Verification items for this drawing (mm, ordinates from the low corner). Round coordinates to 2 decimals unless told otherwise and drop trailing zeros. Loops run counter-clockwise (first coordinate to the right, second up) from the corner with the lowest first, then second, coordinate; pieces in that order, holes last. Notation, with made-up numbers: M -4.75,27 L 1.25,27 A25 ccw 1.25,59 Z; hole C 1,-40 d11. An arc over 180 degrees is marked long. Answer as CSV lines item,"result".
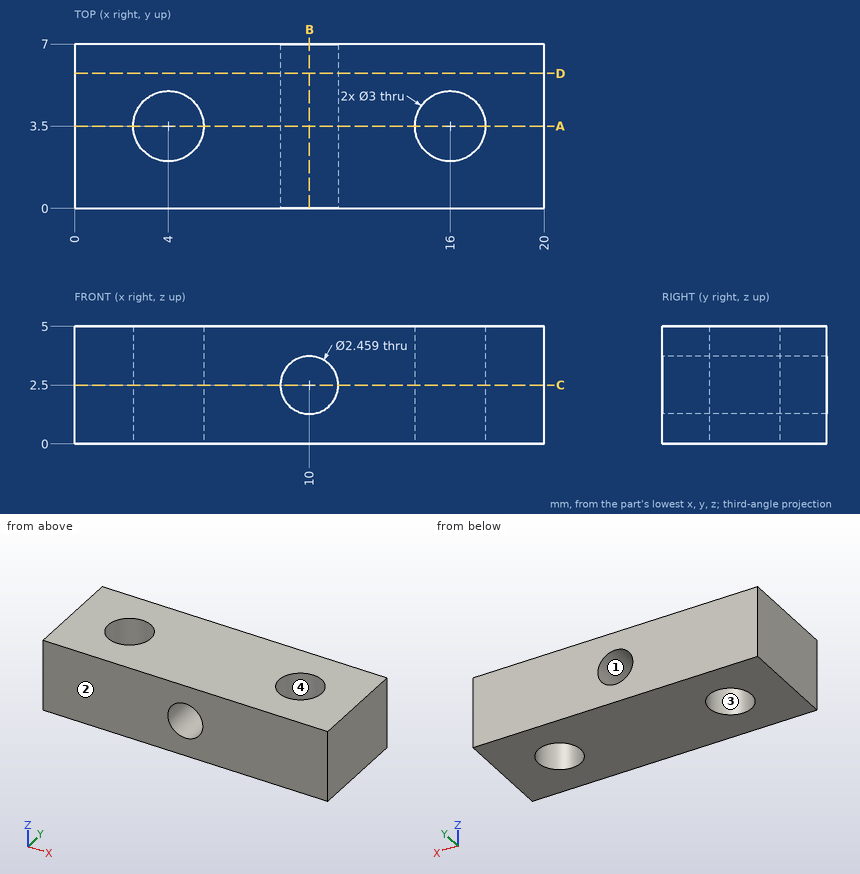
1) Section check D-D (y = 5.75). Record the cut outline in (x, z).
Here are the results:
outline,"M 0,0 L 20,0 L 20,5 L 0,5 Z; hole C 10,2.5 d2.46"
2) Draft check along Y on the marked faces 1, 2, 3 and 4. Enter one of: +Y half, -Y half, draft (parallel to the pull), parting line (faces both ways), or undercut.
Here are the results:
face 1,"draft"
face 2,"-Y half"
face 3,"undercut"
face 4,"undercut"
3) Section check C-C (z = 2.5). Record the cut outline in (x, y).
Here are the results:
outline,"M 0,0 L 8.77,0 L 8.77,7 L 0,7 Z; M 11.23,0 L 20,0 L 20,7 L 11.23,7 Z; hole C 4,3.5 d3; hole C 16,3.5 d3"
4) Material ranges on probe 1 along X at (y, z) = (4.5, 2.5); probe 2 along Y at (x, z) = (4, 3.4); probe 3 along Z at (x, y) = (10, 2.5), recorded low to high.
Here are the results:
probe 1,"x = 0 to 2.88, 5.12 to 8.77, 11.23 to 14.88, 17.12 to 20"
probe 2,"y = 0 to 2, 5 to 7"
probe 3,"z = 0 to 1.27, 3.73 to 5"
5) Section check B-B (x = 10). Record the cut outline in (y, z), plus the area to 3 significant figures.
Here are the results:
outline,"M 0,0 L 7,0 L 7,1.27 L 0,1.27 Z; M 0,3.73 L 7,3.73 L 7,5 L 0,5 Z"
area,"17.8 mm^2"
6) Section check A-A (y = 3.5). Record the cut outline in (x, z), plus the area to 3 significant figures.
Here are the results:
outline,"M 0,0 L 2.5,0 L 2.5,5 L 0,5 Z; M 5.5,0 L 14.5,0 L 14.5,5 L 5.5,5 Z; M 17.5,0 L 20,0 L 20,5 L 17.5,5 Z; hole C 10,2.5 d2.46"
area,"65.3 mm^2"
